Model file for the job. Use its own axes, mm. Round coordinates to 2 decimals unless told otherwise and drop trailing zeros. Order: outer loops, then holes, each group sorted by start corner. A loop starts at its lowest first (then second) coordinate and runs counter-clockwise, first axis right, second up. Notation, with made-up numbers: (38.25, 45) -> (44.25, 45) arc R32 cw to (44.25, 74) -> close; hole circle Ø1 at (49.25, 81.25). An arc over 180 degrees is marked (long way). Answer as CSV lines item,"result".
```python
from build123d import *

# Parameters (mm, degrees)
SKETCH015_R   = 1.5
SKETCH015_R_2 = 2.6
PAD026_DEPTH  = 5
PAD033_DEPTH  = 5
FILLET004_R   = 5


with BuildPart() as part:
    # Sketch015 (on Face1 of Binder015) → Pad026 (new body)
    with BuildSketch(Plane(origin=(-223, 0, 0), x_dir=(0, -1, 0), z_dir=(-1, 0, 0))):
        with BuildLine():
            Line((-21.15, -85), (-21.15, -88))
            ThreePointArc((-21.15, -88), (-16.65, -92.5), (-12.15, -88))
            Line((-12.15, -88), (-12.15, -85))
            Line((-12.15, -85), (12.15, -85))
            Line((12.15, -85), (12.15, -88))
            ThreePointArc((12.15, -88), (16.65, -92.5), (21.15, -88))
            Line((21.15, -88), (21.15, -85))
            Line((21.15, -85), (21.15, 17.6144660941))
            Line((17.6144660941, 21.15), (21.15, 17.6144660941))
            Line((-17.6144660941, 21.15), (17.6144660941, 21.15))
            Line((-21.15, 17.6144660941), (-17.6144660941, 21.15))
            Line((-21.15, 17.6144660941), (-21.15, -85))
        make_face()
        with Locations((16.65, -88)):
            Circle(SKETCH015_R, mode=Mode.SUBTRACT)
        with Locations((-16.65, -88)):
            Circle(SKETCH015_R, mode=Mode.SUBTRACT)
        Circle(SKETCH015_R_2, mode=Mode.SUBTRACT)
    extrude(amount=PAD026_DEPTH)

    # Sketch083 (on DatumPlane) → Pad033 (join, symmetric)
    with BuildSketch(Plane(origin=(-224.6666666667, 0, -49.6166666667), x_dir=(1, 0, 0), z_dir=(0, -1, 0))):
        Polygon((1.6666666667, 36.6166666667), (4.6666666667, 33.6166666667), (4.6666666667, -27.3833333333), (1.6666666667, -30.3833333333), align=None)
    extrude(amount=PAD033_DEPTH, both=True)

    # Fillet004
    fillet004_edges = [part.edges().sort_by_distance(p)[0] for p in [
        (-220, 0, -16),
        (-220, 0, -77),
    ]]
    fillet(fillet004_edges, radius=FILLET004_R)


solid = part.part
```
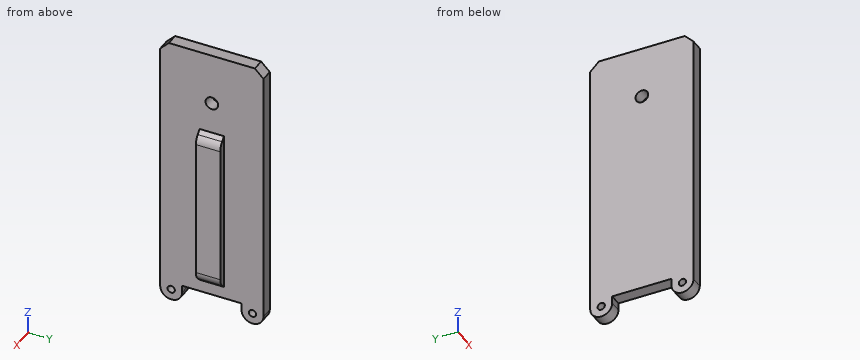
Q1. Saw through at C-C (z = 0). Write the cut outline in (x, y).
Checks:
outline,"(-228, -21.15) -> (-223, -21.15) -> (-223, -2.6) -> (-228, -2.6) -> close; (-228, 2.6) -> (-223, 2.6) -> (-223, 21.15) -> (-228, 21.15) -> close"
Q2. Wall check: L1, parallel to Y at x = -225.25, z = -88; L2, parallel to Z at x = -224.9, y = -16.65; L3, parallel to Z at x = -224.6, y = 0. Give the ranges that are in metal, low to high. Write a range as [from, to].
Checks:
L1,"[-21.15, -18.15], [-15.15, -12.15], [12.15, 15.15], [18.15, 21.15]"
L2,"[-92.5, -89.5], [-86.5, 21.15]"
L3,"[-85, -2.6], [2.6, 21.15]"
Q3. Flat gauge pins, fed straight in: pin 1 (2 mm diameter, centred on x = -227, y = 2.5, fed in from -Z); pin 2 (2 mm diameter, centred on x = -221.5, z = -16, fed in from +Y); pin 3 (5 mm diameter, centred on y = -16.65, z = -88, fed in from +X); pin 4 (4 mm diameter, centred on y = 0, z = 0, fed in from +X). Where does each tip first touch, or does it go through?
Checks:
pin 1,"z = -85"
pin 2,"y = 5"
pin 3,"x = -223"
pin 4,"through"
Q4. Saw through at A-A (x = -227). Write the cut outline in (y, z).
Checks:
outline,"(-21.15, -88) arc R4.5 ccw to (-12.15, -88) -> (-12.15, -85) -> (12.15, -85) -> (12.15, -88) arc R4.5 ccw to (21.15, -88) -> (21.15, 17.61) -> (17.61, 21.15) -> (-17.61, 21.15) -> (-21.15, 17.61) -> close; hole circle Ø3 at (-16.65, -88); hole circle Ø5.2 at (0, 0); hole circle Ø3 at (16.65, -88)"
Q5. Saw through at D-D (z = -51.5). Write the cut outline in (x, y).
Checks:
outline,"(-228, -21.15) -> (-223, -21.15) -> (-223, -5) -> (-220, -5) -> (-220, 5) -> (-223, 5) -> (-223, 21.15) -> (-228, 21.15) -> close"
Q6. Saw through at B-B (y = 0). Write the cut outline in (x, z).
Checks:
outline,"(-228, -85) -> (-223, -85) -> (-223, -80) -> (-221.46, -78.46) arc R5 ccw to (-220, -74.93) -> (-220, -18.07) arc R5 ccw to (-221.46, -14.54) -> (-223, -13) -> (-223, -2.6) -> (-228, -2.6) -> close; (-228, 2.6) -> (-223, 2.6) -> (-223, 21.15) -> (-228, 21.15) -> close"
